```python
from build123d import *

# Parameters (mm, degrees)
F0_R      = 6.35
F1_DEPTH  = 6.35
F2_W      = 6.35
F2_H      = 85.852
F3_DEPTH  = 38.1
F4_W      = 76.2
F4_H      = 9.652
F5_DEPTH  = 76.2
F7_DEPTH  = 10.16
F9_DEPTH  = 9.652
F11_DEPTH = 9.652


with BuildPart() as f1:
    # F0 (on Top) → F1 (new body)
    with BuildSketch(Plane.XY):
        Polygon((0, -85.852), (0, 0), (-38.1, 0), (-76.2, 0), (-76.2, -85.852), align=None)
        with Locations((-38.1, -42.926)):
            Circle(F0_R, mode=Mode.SUBTRACT)
    extrude(amount=F1_DEPTH)

    # F2 (on face) → F3 (join)
    with BuildSketch(Plane(origin=(0, 0, 0), x_dir=(1, 0, 0), z_dir=(0, 0, -1))):
        with Locations((-73.025, 42.926)):
            Rectangle(F2_W, F2_H)
    extrude(amount=F3_DEPTH)

    # F4 (on face) → F5 (join)
    with BuildSketch(Plane(origin=(-76.2, 0, 0), x_dir=(0, -1, 0), z_dir=(-1, 0, 0))):
        with Locations((42.926, -8.128)):
            Rectangle(F4_W, F4_H)
    extrude(amount=F5_DEPTH)

    # F6 (on face) → F7 (cut)
    with BuildSketch(Plane.XY.offset(-3.302)):
        with BuildLine():
            ThreePointArc((-130.041851, -49.243254), (-125.555699, -47.381211), (-123.698, -42.893257))
            ThreePointArc((-123.698, -42.893257), (-125.554284, -38.40672), (-130.037848, -36.543265))
            ThreePointArc((-130.037848, -36.543265), (-136.398, -42.891255), (-130.041851, -49.243254))
        make_face()
        with BuildLine():
            ThreePointArc((-123.698, -42.893257), (-121.838129, -38.40313), (-117.348004, -36.543257))
            Line((-117.348004, -36.543257), (-130.037848, -36.543265))
            ThreePointArc((-130.037848, -36.543265), (-125.554284, -38.40672), (-123.698, -42.893257))
        make_face()
        with BuildLine():
            ThreePointArc((-117.348001, -49.243257), (-112.857872, -47.383386), (-110.998, -42.893257))
            ThreePointArc((-110.998, -42.893257), (-112.857873, -38.403127), (-117.348004, -36.543257))
            ThreePointArc((-117.348004, -36.543257), (-121.838129, -38.40313), (-123.698, -42.893257))
            ThreePointArc((-123.698, -42.893257), (-121.838129, -47.383385), (-117.348001, -49.243257))
        make_face()
        with BuildLine():
            Line((-130.041851, -49.243254), (-117.348001, -49.243257))
            ThreePointArc((-117.348001, -49.243257), (-121.838129, -47.383385), (-123.698, -42.893257))
            ThreePointArc((-123.698, -42.893257), (-125.555699, -47.381211), (-130.041851, -49.243254))
        make_face()
    extrude(amount=-F7_DEPTH, mode=Mode.SUBTRACT)

    # F8 (on face) → F9 (join)
    with BuildSketch(Plane.XZ.offset(81.026)):
        Polygon((-76.2, -12.954), (-152.4, -12.954), (-152.4, -19.304), (-75.782955, -37.925284), align=None)
    extrude(amount=-F9_DEPTH)

    # F10 (on face) → F11 (join)
    with BuildSketch(Plane(origin=(0, -4.826, 0), x_dir=(-1, 0, 0), z_dir=(0, 1, 0))):
        Polygon((152.4, -19.304), (152.4, -12.954), (76.2, -12.954), (75.944759, -37.612777), align=None)
    extrude(amount=-F11_DEPTH)


solid = f1.part
```
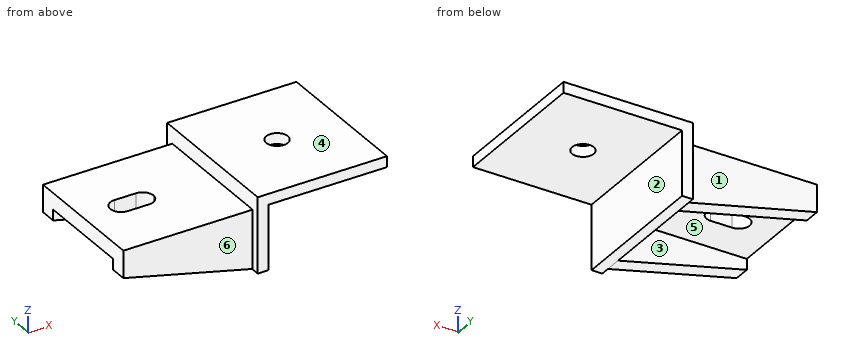
Geometry: final body of the model. Coordinates: model frame, mm. Face numbers are marked on the shaded views. A direction names the side the tool comes from. Give positions to 0.01 mm unless a question says otherwise; leave off trailing zeros. Loops run counter-clockwise (first coordinate to the right, second up) from the corner with the lowest first, then second, coordinate; pieces in that order, holes last. Notation, with made-up numbers: (38, -2) -> (62, -2) arc R25 ccw to (62, 13) -> close; hole circle Ø8 at (83, 85). An arc over 180 degrees is marked (long way). Use one line per item in the form item = value.
Item 1: Section query A-A on z = -5. Output: boundary loops of the cut face in (x, y).
A:
outline = (-152.4, -81.03) -> (-76.2, -81.03) -> (-76.2, -85.85) -> (-69.85, -85.85) -> (-69.85, 0) -> (-76.2, 0) -> (-76.2, -4.83) -> (-152.4, -4.83) -> close; hole (-130.04, -49.24) -> (-117.35, -49.24) arc R6.35 ccw to (-111, -42.89) arc R6.35 ccw to (-117.35, -36.54) -> (-130.04, -36.54) arc R6.35 ccw to start
Item 2: Access query for the marked faces 1, 2 and 3. Directions: +Z, -Z, +X, -X, +Y, -Y. A direction counts if a zero-diameter tool reaches every point of the face in a straight line with its end or side. Return the directions, or none.
A:
face_1 = +Z, -Z, -X, +Y
face_2 = -Z, +X, +Y, -Y
face_3 = -Z, -X
Item 3: Section query B-B on x = -38.1. Output: boundary loops of the cut face in (y, z).
A:
outline = (-85.85, 0) -> (-49.28, 0) -> (-49.28, 6.35) -> (-85.85, 6.35) -> close; (-36.58, 0) -> (0, 0) -> (0, 6.35) -> (-36.58, 6.35) -> close
Item 4: Pin query (flat end, axial travel): P1, Ø12, axis at x = -17, y = -23.5, coming from the -Z side; P2, Ø8, axis at y = -25, z = -22, coming from the +X side; P3, Ø1.5, axis at x = -136.5, z = -19, coming from the +Y side. Return the tip coordinate at first contact, or that it passes through.
A:
P1 = 0
P2 = -69.85
P3 = -4.83
Item 5: Draft query along Y for the marked faces 4, 5 and 6. Return one class per face: pulls with the +Y half, pulls with the -Y half, needs draft (parallel to the pull), parting line crosses it, or undercut.
A:
face_4 = needs draft
face_5 = undercut
face_6 = pulls with the -Y half
Item 6: Line query: probe 1 along Y at (x, z) = (-38, 4); probe 2 along X at (y, z) = (-82, -3.5); probe 3 along Y at (x, z) = (-77, -20.5). Output: solid intervals per line, ascending.
A:
probe_1 = -85.85 to -49.28, -36.58 to 0
probe_2 = -76.2 to -69.85
probe_3 = -81.03 to -71.37, -14.48 to -4.83
Item 7: Section query C-C on y = -34.5. Output: boundary loops of the cut face in (x, z).
A:
outline = (-152.4, -12.95) -> (-76.2, -12.95) -> (-76.2, -38.1) -> (-69.85, -38.1) -> (-69.85, 0) -> (0, 0) -> (0, 6.35) -> (-76.2, 6.35) -> (-76.2, -3.3) -> (-152.4, -3.3) -> close
Item 8: Section query D-D on z = -32. Output: boundary loops of the cut face in (x, y).
A:
outline = (-100.16, -81.03) -> (-76.2, -81.03) -> (-76.2, -85.85) -> (-69.85, -85.85) -> (-69.85, 0) -> (-76.2, 0) -> (-76.2, -4.83) -> (-99.38, -4.83) -> (-99.38, -14.48) -> (-76.2, -14.48) -> (-76.2, -71.37) -> (-100.16, -71.37) -> close
